Read the model definition and answer for the solid it produces. Units are mm, in the model's axes. Coordinates: 2 decimals unless noted, no trailing zeros. Loops run counter-clockwise (first coordinate to the right, second up) from the corner with the lowest first, then second, coordinate; pieces in that order, holes last. Notation, with made-up numbers: (16.5, 55.5) -> (73.5, 55.5) arc R10 ccw to (73.5, 72.5) -> close; hole circle Ø3 at (1.25, 22.25). An arc over 180 degrees is marked (long way). Answer as a JSON object with one key per item and string values. Group by question number.
1) Section C-C, the plane z = -139.7 is taken. Give the vertices of the cut face in (x, y) (1 decimal), plus the area to 3 significant figures.
2) A flat-ended cylindrical pin translates along its axis: P1, Ø12, axis at x = -4.5, y = -20, coming from the +Z side. Find the tip coordinate at first contact, or state that the pin passes through.
3) Section A-A, the plane x = 0.5 is taken. Give the vertices of the cut face in (y, z).
4) Section B-B, the plane z = 4 is taken. Give the vertices of the cut face in (x, y), plus the area to 3 significant figures.
5) Consider probe 1 along Y at (x, z) = (11.65, 152.4); probe 2 along X at (y, z) = (-3, -7); probe 3 along Y at (x, z) = (2, -127). Determine where each line is inside the solid, lowest interval first. Write a range as [from, to].
Autodesk Inventor part; units mm, degrees
ref_plane "YZ Plane" through (0, 0, 0) normal (1, 0, 0) x (0, 1, 0)
ref_plane "XZ Plane" through (0, 0, 0) normal (0, 1, 0) x (-1, 0, 0)
ref_plane "XY Plane" through (0, 0, 0) normal (0, 0, 1) x (1, 0, 0)
sketch "Sketch1" plane through (0, 0, 0) normal (0, 0, 1) x (1, 0, 0)
  line L0 (-12.7, -25.4) -> (12.7, -25.4)
  line L1 (12.7, -25.4) -> (12.7, 25.4)
  line L2 (12.7, 25.4) -> (-12.7, 25.4)
  line L3 (-12.7, 25.4) -> (-12.7, -25.4)
  line L4 (-12.7, -25.4) -> (12.7, 25.4) construction
  line L5 (12.7, -25.4) -> (-12.7, 25.4) construction
  line L6 (-11.1125, 23.8125) -> (11.1125, 23.8125)
  line L7 (11.1125, 23.8125) -> (11.1125, -23.8125)
  line L8 (11.1125, -23.8125) -> (-11.1125, -23.8125)
  line L9 (-11.1125, -23.8125) -> (-11.1125, 23.8125)
  point P0 (0, 0)
  dimension "width" = 25.4
  dimension "height" = 50.8
  dimension "thickness" = 1.5875
extrude "Extrusion1" add sketch "Sketch1" along normal mid plane 330.2
sketch "Sketch3" plane through (12.7, -25.4, -165.1) normal (1, 0, 0) x (0, 0, -1)
  circle A0 centre (-25.4, 25.4) radius 15.875
  line L0 (0, 50.8) -> (0, 0)
  point P0 (-165.1, 25.4)
  dimension "d8" = 31.75
  dimension "d9" = 25.4
extrude "Extrusion3" cut sketch "Sketch3" against normal up to surface (1.5875 mm away)
sketch "Sketch4" plane through (12.7, -25.4, 165.1) normal (1, 0, 0) x (0, 0, -1)
  circle A0 centre (304.8, 25.4) radius 15.875 construction
  line L0 (330.2, 50.8) -> (330.2, 0) construction
  line L1 (330.2, 0) -> (0, 0) construction
  line L2 (0, 0) -> (0, 50.8) construction
  line L3 (0, 50.8) -> (330.2, 50.8) construction
  point P0 (165.1, 25.4)
  point P1 (12.7, 25.4)
  point P2 (12.7, 12.7)
  point P3 (12.7, 38.1)
  point P4 (0, 25.4)
  dimension "d12" = 12.7
  dimension "d13" = 12.7
  dimension "d14" = 12.7
hole "Hole1" at (12.7, 0, 152.4) at (12.7, -12.7, 152.4) at (12.7, 12.7, 152.4) direction (-1, 0, 0) diameter 5.1054 end through all
sketch "Sketch6" plane through (-12.7, -25.4, 165.1) normal (-1, 0, 0) x (0, 0, 1)
  line L0 (-330.2, 0) -> (0, 0) construction
  line L1 (0, 0) -> (-152.4, 0) construction
  circle A0 centre (-12.7, 12.7) radius 2.5527 construction
  circle A1 centre (-12.7, 25.4) radius 2.5527 construction
  circle A2 centre (-12.7, 38.1) radius 2.5527 construction
  line L2 (-330.2, 0) -> (-330.2, 50.8) construction
  line L3 (-330.2, 50.8) -> (0, 50.8) construction
  line L4 (0, 50.8) -> (0, 0) construction
  line L5 (0, 0) -> (-330.2, 0) construction
  circle A3 centre (-12.7, 12.7) radius 2.5527 construction
  circle A4 centre (-12.7, 25.4) radius 2.5527 construction
  circle A5 centre (-12.7, 38.1) radius 2.5527 construction
  line L6 (-330.2, 0) -> (-330.2, 50.8) construction
  line L7 (-330.2, 50.8) -> (0, 50.8) construction
  line L8 (0, 50.8) -> (0, 0) construction
  line L9 (0, 0) -> (-330.2, 0) construction
  line L10 (-152.4, 0) -> (-50.8, 146.1832) construction
  line L11 (0, 0) -> (0, 203.2) construction
  line L12 (0, 203.2) -> (-50.8, 203.2) construction
  line L13 (-50.8, 203.2) -> (-50.8, 146.1832) construction
  circle A6 centre (-106.0668, 44.4119) radius 4.8006 construction
  circle A7 centre (-132.494, 6.3881) radius 4.8006 construction
  line L14 (-106.0668, 44.4119) -> (-132.494, 6.3881) construction
  circle A8 centre (-12.7, 12.7) radius 2.5527 construction
  circle A9 centre (-12.7, 25.4) radius 2.5527 construction
  circle A10 centre (-12.7, 38.1) radius 2.5527 construction
  line L15 (-330.2, 0) -> (-330.2, 50.8) construction
  line L16 (-330.2, 50.8) -> (0, 50.8) construction
  line L17 (0, 50.8) -> (0, 0) construction
  line L18 (0, 0) -> (-330.2, 0) construction
  line L19 (0, 1.5875) -> (-330.2, 1.5875) construction
  line L20 (-330.2, 49.2125) -> (0, 49.2125) construction
  point P0 (-165.1, 25.4)
  dimension "d35" = 152.4
  dimension "d36" = 55.2
  dimension "d37" = 203.2
  dimension "d38" = 50.8
  dimension "d39" = 9.6012
  dimension "d40" = 12.7
hole "Hole3" at (-12.7, 19.0119, 59.0332) at (-12.7, -19.0119, 32.606) direction (1, 0, 0) diameter 9.525 end through all
sketch "Sketch7" plane through (12.7, -25.4, 165.1) normal (1, 0, 0) x (0, 0, -1)
  circle A0 centre (106.0668, 44.4119) radius 4.7625 construction
  circle A1 centre (132.494, 6.3881) radius 4.7625 construction
  circle A2 centre (12.7, 12.7) radius 2.5527 construction
  circle A3 centre (12.7, 25.4) radius 2.5527 construction
  circle A4 centre (12.7, 38.1) radius 2.5527 construction
  circle A5 centre (304.8, 25.4) radius 15.875 construction
  line L0 (330.2, 50.8) -> (0, 50.8) construction
  line L1 (0, 0) -> (0, 50.8) construction
  line L2 (330.2, 0) -> (0, 0) construction
  line L3 (330.2, 50.8) -> (330.2, 0) construction
  line L4 (0, 1.5875) -> (330.2, 1.5875) construction
  line L5 (0, 49.2125) -> (330.2, 49.2125) construction
  line L6 (0, 50.8) -> (152.4, 50.8) construction
  line L7 (330.2, 50.8) -> (0, 50.8) construction
  line L8 (0, 50.8) -> (0, -152.4) construction
  line L9 (0, -152.4) -> (50.8, -152.4) construction
  line L10 (50.8, -152.4) -> (50.8, -95.3832) construction
  line L11 (152.4, 50.8) -> (50.8, -95.3832) construction
  circle A6 centre (132.494, 44.4119) radius 4.8006 construction
  circle A7 centre (106.0668, 6.3881) radius 4.8006 construction
  line L12 (106.0668, 6.3881) -> (132.494, 44.4119) construction
  point P0 (165.1, 25.4)
  dimension "d48" = 152.4
  dimension "d49" = 203.2
  dimension "d50" = 50.8
  dimension "d51" = 55.2
  dimension "d52" = 9.6012
  dimension "d53" = 12.7
hole "Hole4" at (12.7, -19.0119, 59.0332) at (12.7, 19.0119, 32.606) direction (-1, 0, 0) diameter 9.525 end through all
properties part number "CL3-003" material "Aluminum 6061"
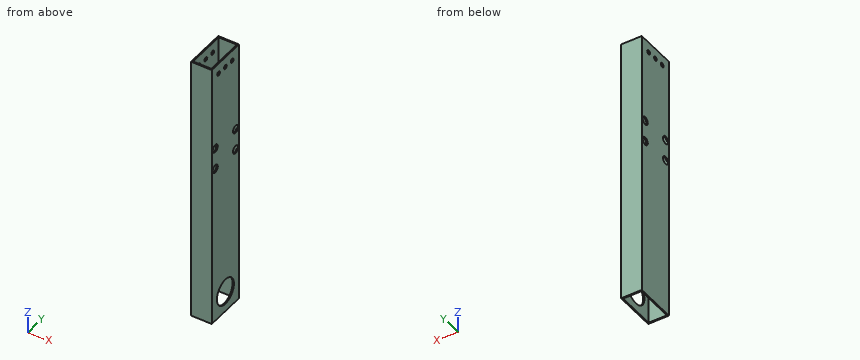
Determined:
{
 "1": {"outline": "(-12.7, -25.4) -> (12.7, -25.4) -> (12.7, -15.9) -> (11.1, -15.9) -> (11.1, -23.8) -> (-11.1, -23.8) -> (-11.1, 23.8) -> (11.1, 23.8) -> (11.1, 15.9) -> (12.7, 15.9) -> (12.7, 25.4) -> (-12.7, 25.4) -> close", "area": "181 mm²"},
 "2": {"P1": "z = 165.1"},
 "3": {"outline": "(-25.4, -165.1) -> (-23.81, -165.1) -> (-23.81, 165.1) -> (-25.4, 165.1) -> close; (23.81, -165.1) -> (25.4, -165.1) -> (25.4, 165.1) -> (23.81, 165.1) -> close"},
 "4": {"outline": "(-12.7, -25.4) -> (12.7, -25.4) -> (12.7, 25.4) -> (-12.7, 25.4) -> close; hole (-11.11, -23.81) -> (11.11, -23.81) -> (11.11, 23.81) -> (-11.11, 23.81) -> close", "area": "232 mm²"},
 "5": {"probe 1": "[-25.4, -15.25], [-10.15, -2.55], [2.55, 10.15], [15.25, 25.4]", "probe 2": "[-12.7, -11.11], [11.11, 12.7]", "probe 3": "[-25.4, -23.81], [23.81, 25.4]"}
}
